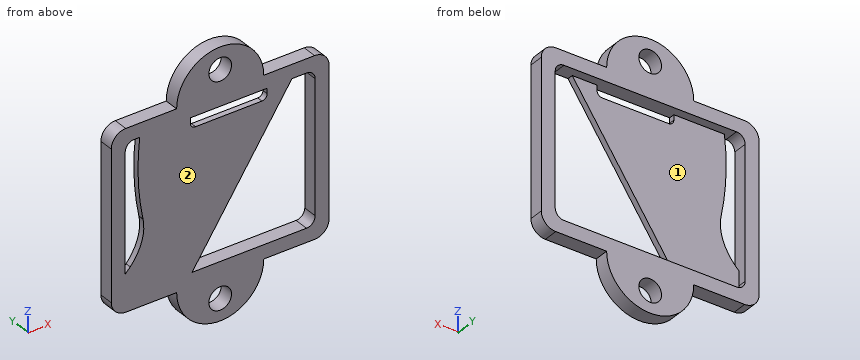
```python
from build123d import *

# Parameters (mm, degrees)
SKETCH1_R           = 3.9
BOSS_EXTRUDE1_DEPTH = 5
CUT_EXTRUDE1_DEPTH  = 3
CUT_EXTRUDE2_DEPTH  = 3
FILLET1_R           = 5
FILLET2_R           = 3


with BuildPart() as part:
    # Sketch1 → Boss-Extrude1 (new body)
    with BuildSketch(Plane(origin=(0, 0, 0), x_dir=(1, 0, 0), z_dir=(0, 1, 0))):
        with BuildLine():
            ThreePointArc((-22.5, 61), (-37.5, 76), (-52.5, 61))
            Line((-52.5, 61), (-75, 61))
            Line((-75, 61), (-75, 0))
            Line((-75, 0), (-52.5, 0))
            ThreePointArc((-52.5, 0), (-37.5, -15), (-22.5, 0))
            Line((-22.5, 0), (0, 0))
            Line((0, 0), (0, 61))
            Line((0, 61), (-22.5, 61))
        make_face()
        with Locations((-37.5, 68.5)):
            Circle(SKETCH1_R, mode=Mode.SUBTRACT)
        with Locations((-37.5, -7.5)):
            Circle(SKETCH1_R, mode=Mode.SUBTRACT)
    extrude(amount=BOSS_EXTRUDE1_DEPTH)

    # Sketch2 → Cut-Extrude1 (cut)
    with BuildSketch(Plane(origin=(0, 5, 0), x_dir=(1, 0, 0), z_dir=(0, 1, 0))):
        Polygon((-5.840163934, 4.75), (-69.159836066, 56.25), (-70.2, 56.25), (-70.2, 4.75), align=None)
        Polygon((-4.8, 56.25), (-69.159836066, 56.25), (-5.840163934, 4.75), (-4.8, 4.75), align=None)
    extrude(amount=-CUT_EXTRUDE1_DEPTH, mode=Mode.SUBTRACT)

    # Sketch3 → Cut-Extrude2 (cut, through all)
    with BuildSketch(Plane(origin=(0, 2, 0), x_dir=(1, 0, 0), z_dir=(0, 1, 0))):
        with BuildLine():
            add(Edge.make_bspline(
                [(-70.2, 48.25), (-69.3360202, 47.393408535), (-68.484165296, 46.526885218)],
                knots=[0, 0, 0, 0.044512792, 0.044512792, 0.044512792], degree=2))
            Line((-70.2, 48.25), (-70.2, 4.75))
            Line((-70.2, 4.75), (-65.2, 4.75))
            add(Edge.make_bspline(
                [(-65.2, 4.75), (-66.281505433, 14.095378491), (-65.909161294, 23.268767529), (-64.082967584, 32.270167116)],
                knots=[0, 0, 0, 0, 0.780709758, 0.780709758, 0.780709758, 0.780709758], degree=3))
            add(Edge.make_bspline(
                [(-64.082967584, 32.270167116), (-64.075541276, 32.30677176), (-64.068090925, 32.343373559), (-64.060616532, 32.379972514)],
                knots=[0.780709758, 0.780709758, 0.780709758, 0.780709758, 0.783884554, 0.783884554, 0.783884554, 0.783884554], degree=3))
            add(Edge.make_bspline(
                [(-68.484165296, 46.526885218), (-65.083389168, 42.682237292), (-63.043469729, 37.485478449), (-64.060616531, 32.379972514)],
                knots=[0.136165996, 0.136165996, 0.136165996, 0.136165996, 0.993850371, 0.993850371, 0.993850371, 0.993850371], degree=3))
        make_face()
        Polygon((-12.8, 56.25), (-47.2, 56.25), (-12.8, 4.75), (-4.8, 4.75), (-4.8, 56.25), align=None)
        with BuildLine():
            Line((-23.141162666, 4.75), (-21.341162666, 4.75))
            Line((-21.341162666, 4.75), (-21.341162666, 6.55))
            ThreePointArc((-21.341162666, 6.55), (-21.86837046, 7.822792206), (-23.141162666, 8.35))
            Line((-23.141162666, 8.35), (-45.995816889, 8.35))
            ThreePointArc((-45.995816889, 8.35), (-47.268609095, 7.822792206), (-47.795816889, 6.55))
            Line((-47.795816889, 6.55), (-47.795816889, 4.75))
            Line((-47.795816889, 4.75), (-45.995816889, 4.75))
            Line((-45.995816889, 4.75), (-23.141162666, 4.75))
        make_face()
    extrude(amount=-CUT_EXTRUDE2_DEPTH, mode=Mode.SUBTRACT)

    # Fillet1
    fillet1_edges = [part.edges().sort_by_distance(p)[0] for p in [
        (-75, 2.5, -61),
        (0, 2.5, -61),
        (0, 2.5, 0),
        (-75, 2.5, 0),
    ]]
    fillet(fillet1_edges, radius=FILLET1_R)

    # Fillet2
    fillet2_edges = [part.edges().sort_by_distance(p)[0] for p in [
        (-70.2, 3.5, -56.25),
        (-4.8, 2.5, -56.25),
        (-4.8, 2.5, -4.75),
        (-70.2, 2.5, -4.75),
    ]]
    fillet(fillet2_edges, radius=FILLET2_R)


solid = part.part
```
Read the model definition and answer for the solid it produces. Units are mm, in the model's axes. Face numbers are marked on the shaded views. Round coordinates to 2 decimals unless told otherwise and drop trailing zeros. Write each loop counter-clockwise with the first axis right and the second up, starting at its lowest first coordinate (ties: lowest second). Pieces come first, ordered by that corner, then holes. Notation, with made-up numbers: (85.25, -22.5) - (112.25, -22.5) arc R18 cw to (112.25, -17.5) - close; hole circle Ø11 at (22.25, 33). An arc over 180 degrees is marked (long way). One line per item, written item: value.
Q1. For a pull along Z with two mould halves and no side action, classify the marked faces 1 and 2 as pulls with the +Z half, pulls with the -Z half, needs draft (parallel to the pull), parting line crosses it, or undercut.
The answers:
face 1: undercut
face 2: needs draft
Q2. Straight lines are drawn through the part: line 1 (Z direction, x = -37.5, y = 2.35); line 2 (X direction, y = 4.5, z = -32); line 3 (Z direction, x = -53, y = 3.05). For each, find the intervals that lie inside material, in ascending order. Write a range as from..to.
The answers:
line 1: z = -76..-72.4, -64.6..-56.25, -4.75..3.6, 11.4..15
line 2: x = -75..-70.2, -4.8..0
line 3: z = -61..-56.25, -4.75..0
Q3. Find section B-B (z = -68.5). Determine the outline of the cut face in (x, y), and give its area (3 significant figures).
The answers:
outline: (-50.49, 0) - (-41.4, 0) - (-41.4, 5) - (-50.49, 5) - close; (-33.6, 0) - (-24.51, 0) - (-24.51, 5) - (-33.6, 5) - close
area: 90.9 mm2
Q4. Each of these flat-tipped pins is pushed along its axis until it touches: P1, Ø1.5, axis at y = 1.5, z = -3.5, coming from the -X side; P2, Ø6, axis at x = -37.5, z = 7.5, coming from the +Y side; P3, Ø1.5, axis at x = -10.5, y = 2.5, coming from the -Z side; P4, Ø12, axis at x = -55, z = -13, coming from the +Y side. Where does it stop, or does it pass through?
The answers:
P1: stops at x = -74.94
P2: passes through
P3: stops at z = -61
P4: stops at y = 2
Q5. Find section D-D (z = -28.5). Count the separate pieces of the cut face and the enclosed holes in it, and give its area (3 significant figures).
The answers:
separate pieces: 3
enclosed holes: 0
area: 120 mm2
Q6. Find section A-A (y = 3.4). Determine the outline of the cut face in (x, z).
The answers:
outline: (-75, -56) arc R5 ccw to (-70, -61) - (-52.5, -61) arc R15 ccw to (-22.5, -61) - (-5, -61) arc R5 ccw to (0, -56) - (0, -5) arc R5 ccw to (-5, 0) - (-22.5, 0) arc R15 ccw to (-52.5, 0) - (-70, 0) arc R5 ccw to (-75, -5) - close; hole (-70.2, -53.25) arc R3 ccw to (-67.2, -56.25) - (-7.8, -56.25) arc R3 ccw to (-4.8, -53.25) - (-4.8, -7.75) arc R3 ccw to (-7.8, -4.75) - (-67.2, -4.75) arc R3 ccw to (-70.2, -7.75) - close; hole circle Ø7.8 at (-37.5, -68.5); hole circle Ø7.8 at (-37.5, 7.5)
Q7. Find section C-C (z = -59). Determine the outline of the cut face in (x, y), and give its area (3 significant figures).
The answers:
outline: (-74, 0) - (-1, 0) - (-1, 5) - (-74, 5) - close
area: 365 mm2
